Check sheet for the modelled part. Datum: model origin and axes. Units: mm. Coordinates: 2 decimals unless noted, no trailing zeros. Write each loop counter-clockwise with the first axis right and the second up, starting at its lowest first coordinate (ties: lowest second). Pieces come first, ordered by that corner, then holes. Notation, with made-up numbers: M -33.5,68.25 L 7.5,68.25 A23 ccw 7.5,107.25 Z; hole C 19.25,57.25 d4. An arc over 180 degrees is marked long. Answer as CSV lines item,"result". Start each with the question number.
Q1. Sectioned sample at A-A, the plane y = 0.8. Record the cut outline in (x, z), then the cut area to 3 significant figures.
Q2. Depth check by flat-ended pin: pin 1 Ø2.5 at (x, z) = (0, 10) entering from -Y. Enter the tip coordinate at first touch or a pass-through.
Q3. Sectioned sample at B-B, the plane z = 115. Record the cut outline in (x, y), then the cut area to 3 significant figures.
Q4. Thickness scan on line 1 along Z through (x, y) = (-3.5, 0); line 2 along X through (y, z) = (0.7, 20); line 3 along Z through (x, y) = (4.25, 1.2). Record the ranges inside material, lowest first. Write a range as from..to.
Solid Edge part; units mm, degrees
sketch "Sketch1" plane through (0, 0, 0) normal (0, 0, 1) x (1, 0, 0)
  line L0 (-10, -1.5) -> (10, -1.5)
  line L1 (10, -1.5) -> (10, 1.5)
  line L2 (10, 1.5) -> (-10, 1.5)
  line L3 (-10, 1.5) -> (-10, -1.5)
  dimension "D1" = 10
  dimension "D2" = 10
  dimension "D3" = 10
extrude "Protrusion1" add sketch "Sketch1" along normal blind 390
sketch "Sketch2" plane through (0, -1.5, 157.5) normal (0, -1, 0) x (0, 0, -1)
  circle A0 centre (-212.5, 0) radius 1.5
  circle A1 centre (137.5, 0) radius 1.5
  circle A2 centre (147.5, 0) radius 1.5
  circle A3 centre (-222.5, 0) radius 1.5
  dimension "D1" = 137.5
extrude "ExtrudedCutout_1" cut sketch "Sketch2" along normal mid plane 784.3163
sketch "Sketch3" plane through (0, -1.5, 157.5) normal (0, -1, 0) x (0, 0, -1)
  line L0 (-112.5, -10) -> (-122.5, -10)
  line L1 (-122.5, -10) -> (-122.5, 0)
  line L2 (-112.5, 0) -> (-112.5, -10)
  arc A0 (-122.5, 0) -> (-112.5, 0) centre (-117.5, 0) cw
  line L3 (47.5, 0) -> (47.5, -10)
  line L4 (47.5, -10) -> (37.5, -10)
  line L5 (37.5, -10) -> (37.5, 0)
  arc A1 (47.5, 0) -> (37.5, 0) centre (42.5, 0) ccw
  dimension "D1" = 112.5
  dimension "D2" = 37.5
extrude "ExtrudedCutout_2" cut sketch "Sketch3" against normal blind 359.7683
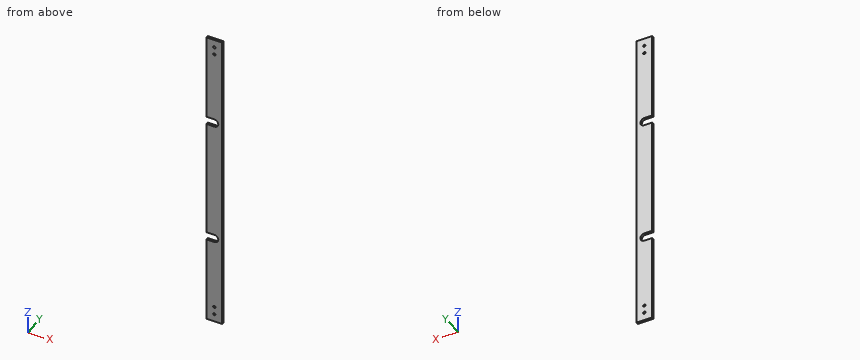
Output:
1,outline,"M -10,0 L 10,0 L 10,390 L -10,390 L -10,280 L 0,280 A5 cw 0,270 L -10,270 L -10,120 L 0,120 A5 cw 0,110 L -10,110 Z; hole C 0,10 d3; hole C 0,20 d3; hole C 0,370 d3; hole C 0,380 d3"
1,area,"7,490 mm^2"
2,pin 1,"passes through"
3,outline,"M 5,-1.5 L 10,-1.5 L 10,1.5 L 5,1.5 Z"
3,area,"15.0 mm^2"
4,line 1,"z = 0..110, 120..270, 280..390"
4,line 2,"x = -10..-1.5, 1.5..10"
4,line 3,"z = 0..112.37, 117.63..272.37, 277.63..390"
